Geometry: see drawing. Coordinates: mm, zero at the bounding-box minimum. Coordinates: 2 decimals unless noted, no trailing zeros.
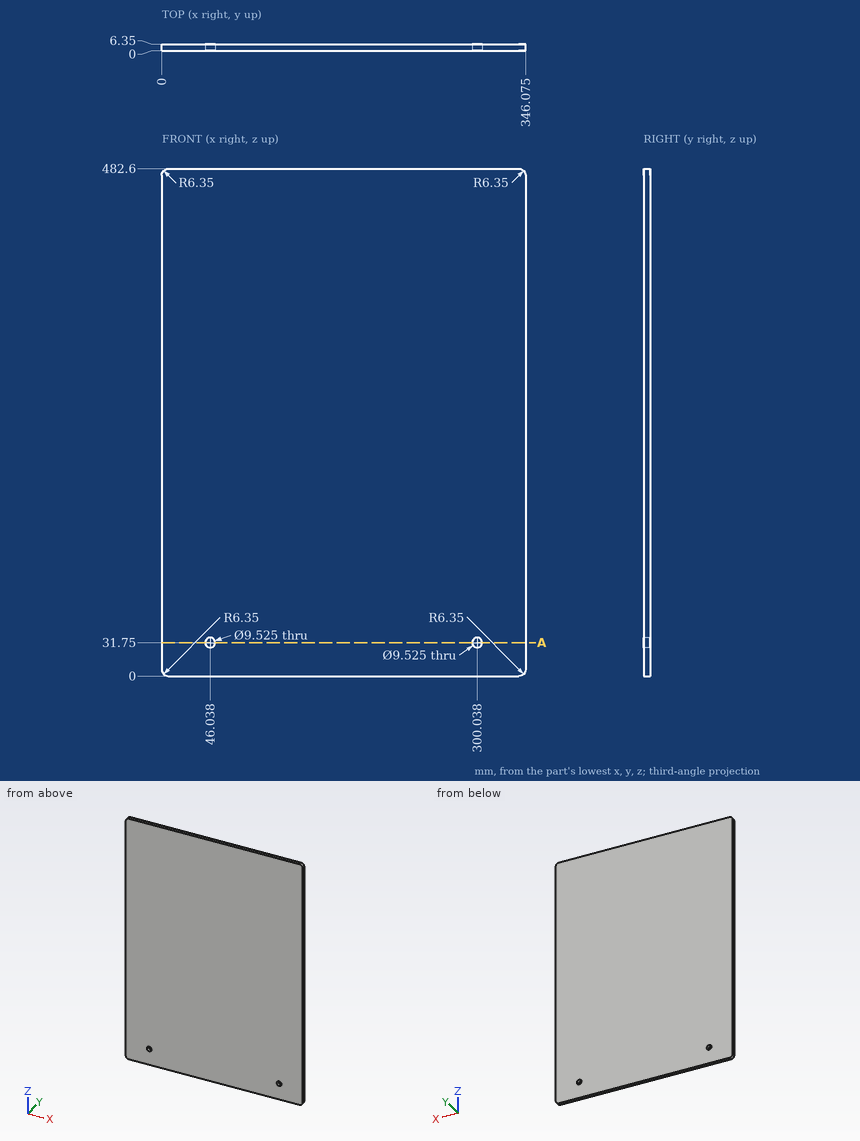
Item 1: Material intervals for probe 1 along X at (y, z) = (1.5, 31.75) (1 decimal); probe 2 along Z at (x, y) = (299, 5.75), sorted ascending.
Derived:
probe 1: x = 0 to 41.3, 50.8 to 295.3, 304.8 to 346.1
probe 2: z = 0 to 27.1, 36.4 to 482.6
Item 2: Pin query (flat end, axial travel): pin 1 (7.5 mm diameter, centred on x = 46.04, z = 31.75, fed in from +Y). Return the tip coordinate at first contact, or that it passes through.
Derived:
pin 1: passes through
Item 3: Section A-A, the plane z = 31.75. State how many separate pieces and enclosed holes the cut face has, plus the area to 3 significant figures.
Derived:
separate pieces: 3
enclosed holes: 0
area: 2,080 mm2
